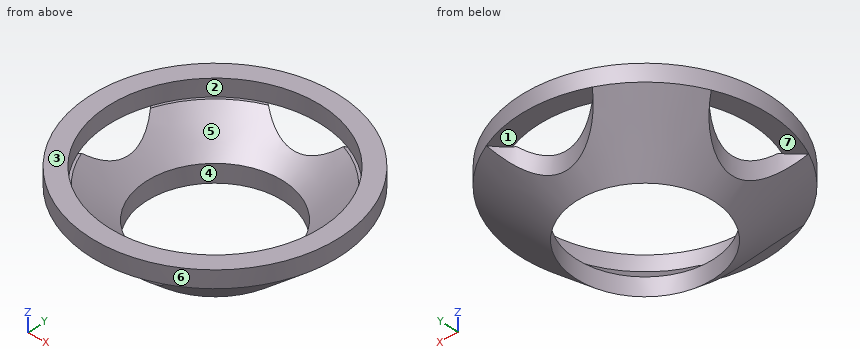
```python
from build123d import *

# Parameters (mm, degrees)
SKETCH1_R           = 13.85
SKETCH1_R_2         = 11.85
BOSS_EXTRUDE1_DEPTH = 1.9
SKETCH4_R           = 7
SKETCH4_R_2         = 7.613586195
CUT_EXTRUDE2_DEPTH  = 5.5


with BuildPart() as part:
    # Sketch1 → Boss-Extrude1 (new body)
    with BuildSketch(Plane.XY):
        with Locations(Location((0, 0, 0), (0, 0, 180))):
            Circle(SKETCH1_R)
        with Locations(Location((0, 0, 0), (0, 0, 180))):
            Circle(SKETCH1_R_2, mode=Mode.SUBTRACT)
    extrude(amount=BOSS_EXTRUDE1_DEPTH)

    # Sketch2 → Revolve1 (revolve)
    with BuildSketch(Plane(origin=(0, 0, 0), x_dir=(1, 0, 0), z_dir=(0, 1, 0))):
        Polygon((-13.85, 0), (-7.613586195, 5.5), (0, 5.5), (0, 3.5), (-7.613586195, 3.5), (-11.582213162, 0), align=None)
    revolve(axis=Axis((0, 0, -5.5), (0, 0, 1)))

    # Sketch4 → Cut-Extrude2 (cut)
    with BuildSketch(Plane(origin=(0, 0, -5.5), x_dir=(-1, 0, 0), z_dir=(0, 0, -1))):
        with Locations((16.5, 0)):
            Circle(SKETCH4_R)
        Circle(SKETCH4_R_2)
        with Locations((0, -16.5)):
            Circle(SKETCH4_R)
        with Locations((0, 16.5)):
            Circle(SKETCH4_R)
    extrude(amount=-CUT_EXTRUDE2_DEPTH, mode=Mode.SUBTRACT)


solid = part.part
```
Check sheet for the modelled part. Datum: model origin and axes. Units: mm. Face numbers are marked on the shaded views. A direction names the side the tool comes from. Give positions to 0.01 mm unless a question says otherwise; leave off trailing zeros. Order: outer loops, then holes, each group sorted by start corner. A loop starts at its lowest first (then second) coordinate and runs counter-clockwise, first axis right, second up. Notation, with made-up numbers: M -1,-7 L 30,-7 A8 ccw 30,1 Z; hole C 68.5,49 d8. An arc over 180 degrees is marked long. Answer in a Markdown table with one row per item. Add a question column.
Q1. Release check for a two-part mould opening along X. For the marked faces 4, 5, 6 and 7 record: released by +X, released by -X, zero draft, split by the parting line, or undercut.
Q2. Gauge pin test, flat ends, axial feed: pin 1 Ø2.5 at (x, y) = (-2.5, -13) entering from -Z; pin 2 Ø4 at (y, z) = (7, -4) entering from +X; pin 3 Ø1.5 at (x, y) = (-3.5, -8.5) entering from -Z. Record the tip position at first contact, or that the pin passes through.
Q3. Sectioned sample at B-B, the plane y = 0. Record the boundary of the cut face in (x, z).
Q4. Sectioned sample at C-C, the plane z = -0.75. Record the boundary of the cut face in (x, y).
Q5. Sectioned sample at A-A, the plane x = 0. Record the boundary of the cut face in (y, z).
Q6. Sectioned sample at D-D, the plane z = -3. Record the boundary of the cut face in (x, y).
Q7. Access from +Z, -Z, +X, -X, +Y, -Y to the whole of each face (thin tool, end or side, straight path). Record for the marked faces 1, 2 and 3.
Q8. Thickness scan on L1, parallel to X at y = 8, z = -2; L2, parallel to Y at x = -0.5, z = -2; L3, parallel to Y at x = -10, z = 0.5. Record the ranges inside material, lowest first.
Verdict:
| question | item | result |
|---|---|---|
| 1 | face 4 | undercut |
| 1 | face 5 | undercut |
| 1 | face 6 | split by the parting line |
| 1 | face 7 | zero draft |
| 2 | pin 1 | z = 0 |
| 2 | pin 2 | x = 9.56 |
| 2 | pin 3 | z = -4.77 |
| 3 | outline | M -13.85,0 L -11.85,0 L -11.85,1.9 L -13.85,1.9 Z; M -9.5,-3.84 L -7.61,-5.5 L -7.61,-3.5 L -9.5,-1.84 Z; M 7.61,-5.5 L 13.85,0 L 13.85,1.9 L 11.85,1.9 L 11.85,0 L 11.58,0 L 7.61,-3.5 Z |
| 4 | outline | M -11.89,-5.26 A13 ccw -5.26,-11.89 A7 cw -3.16,-10.26 A10.73 cw -10.26,-3.16 A7 cw Z; M -11.89,5.26 A7 cw -10.26,3.16 A10.73 cw -3.16,10.26 A7 cw -5.26,11.89 A13 ccw Z; M 3.16,-10.26 A7 cw 5.26,-11.89 A13 ccw 5.26,11.89 A7 cw 3.16,10.26 A10.73 cw Z |
| 5 | outline | M -13.85,0 L -11.85,0 L -11.85,1.9 L -13.85,1.9 Z; M -9.5,-3.84 L -7.61,-5.5 L -7.61,-3.5 L -9.5,-1.84 Z; M 7.61,-5.5 L 9.5,-3.84 L 9.5,-1.84 L 7.61,-3.5 Z; M 11.85,0 L 13.85,0 L 13.85,1.9 L 11.85,1.9 Z |
| 6 | outline | M -10.07,-2.77 A10.45 ccw -2.77,-10.07 A7 cw 2.77,-10.07 A10.45 ccw 2.77,10.07 A7 cw -2.77,10.07 A10.45 ccw -10.07,2.77 A7 cw Z; hole C 0,0 d16.36 |
| 7 | face 1 | -Z, +Y |
| 7 | face 2 | +Z |
| 7 | face 3 | +Z, +X, -X, +Y, -Y |
| 8 | L1 | -8.38 to -4.77, 4.77 to 8.38 |
| 8 | L2 | -9.52 to -9.3, 9.3 to 9.52 |
| 8 | L3 | -9.58 to -6.36, 6.36 to 9.58 |
